Here's the drawing with two shaded views (mm, measured from the low corner). I have some questions. A direction names the side the tool comes from. Coordinates: 2 decimals unless noted, no trailing zeros. Write each loop counter-clockwise with the first axis right and the second up, starting at its lowest first coordinate (ties: lowest second). Pieces come first, ordered by that corner, then holes. Notation, with made-up numbers: (47.5, 52) - (54.5, 52) arc R15 cw to (54.5, 56) - close; hole circle Ø9 at (81.5, 82.25). An arc over 180 degrees is marked (long way). Answer in a Markdown table with one row per item. Add a question column.
Item 1: Which directions (+Z, -Z, +X, -X, +Y, -Y) give clear straight access to the entire face, cutting with the end or side of a thin tool? Please do the marked faces 1 and 2.
Item 2: Imagine slicing it at C-C (y = 9.5). Please give me the cut outline in (x, z).
Item 3: Imagine slicing it at B-B (x = 116). Please give me the cut outline in (y, z), plus the area to 3 significant figures.
Item 4: Imagine slicing it at A-A (z = 116). Please give me the cut outline in (x, y), plus the area to 3 significant figures.
Item 5: I'm going to push flat-ended pins straight in: pin 1 (2 mm diameter, centred on y = 22, z = 91.5, fed in from -X); pin 2 (1.5 mm diameter, centred on x = 101, z = 101.5, fed in from -Y); pin 3 (5 mm diameter, centred on x = 127, y = 70.5, fed in from -Z); pin 4 (3 mm diameter, centred on x = 32.5, z = 57.5, fed in from +Y). Where does each tip first touch, or does it pass through?
Item 6: Imagine slicing it at D-D (x = 70.5). Please give me the cut outline in (y, z), plus the area to 3 significant figures.
Item 7: If I drill on probe 1 along Y at (x, z) = (193.5, 88.5); probe 2 along X at (y, z) = (18, 168.5); probe 3 along X at (y, z) = (7, 25), over which ranges is the centre line in solid material (lowest first)? Write a range as from..to.
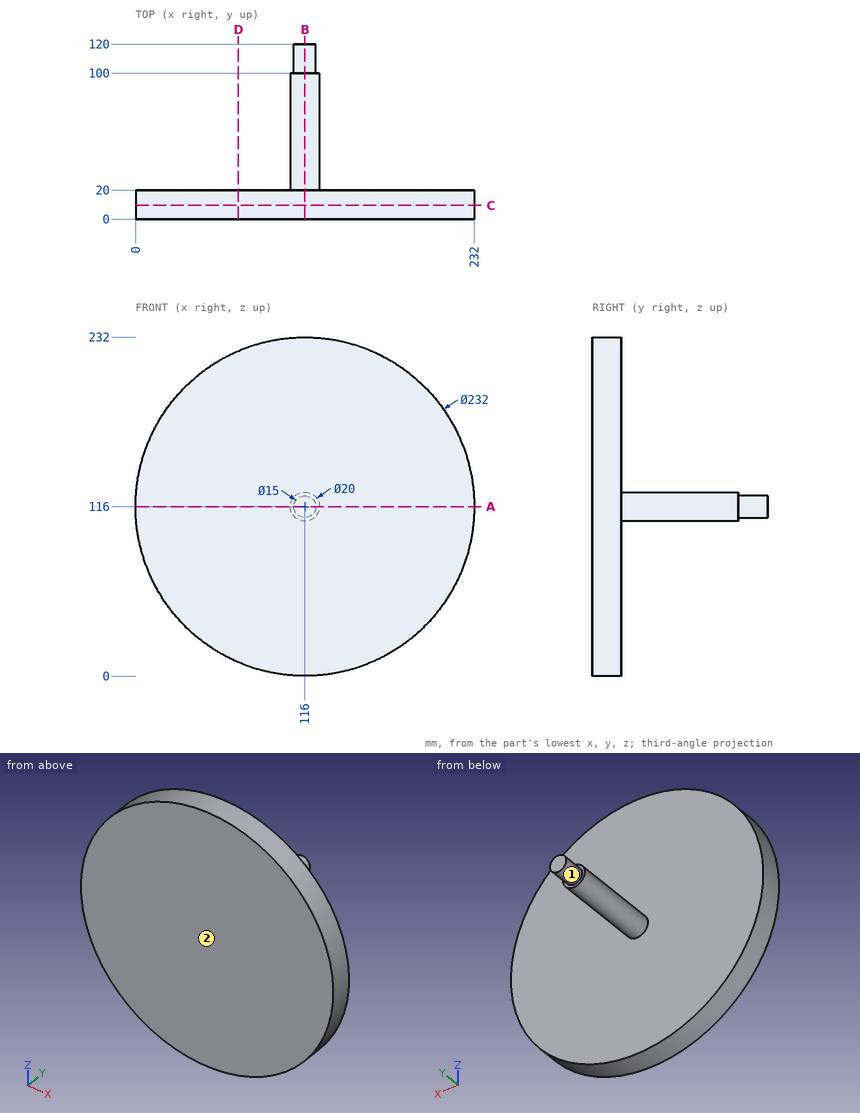
Here are the results:
| question | item | result |
|---|---|---|
| 1 | face 1 | +Y |
| 1 | face 2 | +Z, -Z, +X, -X, -Y |
| 2 | outline | circle Ø232 at (116, 116) |
| 3 | outline | (0, 0) - (20, 0) - (20, 106) - (100, 106) - (100, 108.5) - (120, 108.5) - (120, 123.5) - (100, 123.5) - (100, 126) - (20, 126) - (20, 232) - (0, 232) - close |
| 3 | area | 6,540 mm2 |
| 4 | outline | (0, 0) - (232, 0) - (232, 20) - (126, 20) - (126, 100) - (123.5, 100) - (123.5, 120) - (108.5, 120) - (108.5, 100) - (106, 100) - (106, 20) - (0, 20) - close |
| 4 | area | 6,540 mm2 |
| 5 | pin 1 | passes through |
| 5 | pin 2 | stops at y = 0 |
| 5 | pin 3 | stops at z = 110.73 |
| 5 | pin 4 | stops at y = 20 |
| 6 | outline | (0, 9.3) - (20, 9.3) - (20, 222.7) - (0, 222.7) - close |
| 6 | area | 4,270 mm2 |
| 7 | probe 1 | y = 0..20 |
| 7 | probe 2 | x = 12.56..219.44 |
| 7 | probe 3 | x = 44.06..187.94 |
